Can you work these out from the model? Positions are in its coordinate system, mm. Round coordinates to 2 decimals unless told otherwise and drop trailing zeros. Order: outer loops, then holes, each group sorted by start corner. A loop starts at its lowest first (then second) coordinate and runs counter-clockwise, first axis right, second up. Notation, with made-up numbers: (-33, 29) -> (11, 29) arc R18 cw to (11, 61) -> close; hole circle Ø9 at (-35.75, 55.25). An arc over 180 degrees is marked (long way). Use a Markdown table: item, result. Add a question column.
Q1. I need wall thicknesses on line 1 along Y through (x, z) = (1.85, -261); line 2 along Y through (x, z) = (2.1, -269); line 3 along Z through (x, y) = (1.3, -61.5). Which ranges of each line are inside material? Lowest first, please. Write a range as [from, to].
Q2. If we section it at A-A on x = 1.4: List the corners of the cut face in (y, z) for me, plus the area to 3 significant figures.
Q3. If we section it at B-B on y = 43: List the corners of the cut face in (x, z) for me.
Q4. I'm going to push flat-ended pins straight in: pin 1 Ø1.5 at (x, y) = (1, -55.5) entering from -Z; pin 2 Ø4.5 at (y, z) = (-6.23, -205.18) entering from -X; pin 3 Ø1 at (x, y) = (1, -40) entering from -Z. Where does each tip first touch, or does it pass through?
Q5. If we section it at C-C on z = -256: List the corners of the cut face in (x, y) for me, plus the area to 3 significant figures.
Autodesk Inventor part; units mm, degrees
ref_plane "YZ Plane" through (0, 0, 0) normal (1, 0, 0) x (0, 1, 0)
ref_plane "XZ Plane" through (0, 0, 0) normal (0, 1, 0) x (-1, 0, 0)
ref_plane "XY Plane" through (0, 0, 0) normal (0, 0, 1) x (1, 0, 0)
sketch "スケッチ1" plane through (0, 0, 0) normal (1, 0, 0) x (0, 1, 0)
  line L0 (-90, 103.923) -> (-90, -196.077)
  line L1 (-90, -196.077) -> (90, -300)
  line L2 (-126, 0) -> (126, 0)
  line L3 (0, -380.7846) -> (0, 184.7077)
  line L4 (-90, 103.923) -> (-38.1407, 52.0638)
  line L5 (-38.1407, 52.0638) -> (90, -300)
  dimension "d0" = 300
  dimension "d5" = 90
  dimension "d6" = 300
  dimension "d7" = 90
  dimension "d32" = 20
  dimension "d33" = 40
  dimension "d34" = 45
extrude "押し出し1" add sketch "スケッチ1" along normal blind 3 contours L4 L5 L2 L0 | L2 L5 L3 L1 L0 | L3 L5 L1
fillet "フィレット1" radius 5 1 edges at (1.5, 90, -300)
sketch "スケッチ3" plane through (3, 0, 0) normal (1, 0, 0) x (0, 0, -1)
  circle A0 centre (245.7766, 34.0822) radius 2.5
  line L0 (196.077, -90) -> (293.1313, 78.1031)
  line L1 (287.0911, 85.3015) -> (-52.0638, -38.1407)
  circle A1 centre (205.1793, -6.2342) radius 2.5
  circle A2 centre (174.9758, -22.5483) radius 2.5
  circle A3 centre (89.5158, -22.792) radius 2.5
  line L2 (89.5158, -22.792) -> (174.9758, -22.5483)
  point P0 (0, 0)
  dimension "d36" = 34
  dimension "d37" = 5
  dimension "d38" = 5
  dimension "d40" = 58
  dimension "d41" = 63
  dimension "d42" = 34
  dimension "d43" = 5
  dimension "d44" = 5
  dimension "d45" = 19
  dimension "d46" = 34
  dimension "d47" = 52
  dimension "d51" = 85.46
extrude "押し出し3" cut sketch "スケッチ3" against normal through all
properties part number "stay_middle" material "アルミニウム 6061"
Answer below:
| question | item | result |
|---|---|---|
| 1 | line 1 | [22.45, 75.81] |
| 1 | line 2 | [36.31, 78.72] |
| 1 | line 3 | [-212.53, 75.42] |
| 2 | outline | (-90, -196.08) -> (78.1, -293.13) arc R5 ccw to (85.3, -287.09) -> (-38.14, 52.06) -> (-90, 103.92) -> close; hole circle Ø5 at (-22.79, -89.52); hole circle Ø5 at (-22.55, -174.98); hole circle Ø5 at (-6.23, -205.18); hole circle Ø5 at (34.08, -245.78) |
| 2 | area | 32,700 mm² |
| 3 | outline | (0, -272.86) -> (3, -272.86) -> (3, -170.87) -> (0, -170.87) -> close |
| 4 | pin 1 | z = -216.43 |
| 4 | pin 2 | through |
| 4 | pin 3 | z = -225.23 |
| 5 | outline | (0, 13.79) -> (3, 13.79) -> (3, 73.99) -> (0, 73.99) -> close |
| 5 | area | 181 mm² |
